Autodesk Inventor part; units mm, degrees
ref_plane "YZ Plane" through (0, 0, 0) normal (1, 0, 0) x (0, 1, 0)
ref_plane "XZ Plane" through (0, 0, 0) normal (0, 1, 0) x (-1, 0, 0)
ref_plane "XY Plane" through (0, 0, 0) normal (0, 0, 1) x (1, 0, 0)
sketch "Sketch1" plane through (0, 0, 0) normal (0, 1, 0) x (-1, 0, 0)
  circle A0 centre (0, 0) radius 3.175
  dimension "d0" = 6.35
extrude "Extrusion1" add sketch "Sketch1" along normal blind 31.75
sketch "Sketch2" plane through (0, 31.75, 0) normal (0, 1, 0) x (1, 0, 0)
  circle A0 centre (0, 0) radius 3.175
  circle A1 centre (0, 0) radius 4.7625
  dimension "d3" = 9.525
extrude "Extrusion2" add sketch "Sketch2" along normal blind 6.35 contours A0 | A1
sketch "Sketch3" plane through (0, 38.1, 0) normal (0, 1, 0) x (1, 0, 0)
  circle A0 centre (0, 0) radius 4.7625
  line L0 (-1.3748, 2.3812) -> (1.3748, 2.3813)
  line L1 (1.3748, 2.3813) -> (2.7496, 0)
  line L2 (2.7496, 0) -> (1.3748, -2.3813)
  line L3 (1.3748, -2.3813) -> (-1.3748, -2.3813)
  line L4 (-1.3748, -2.3813) -> (-2.7496, 0)
  line L5 (-2.7496, 0) -> (-1.3748, 2.3812)
  dimension "d6" = 4.7625
extrude "Extrusion3" cut sketch "Sketch3" against normal blind 3.175 contours L0 L1 L2 L3 L4 L5
fillet "Fillet1" radius 0.3969 3 edges at (3.175, 31.75, 0) (-4.7625, 38.1, 0) (3.175, 0, 0)
properties part number "Bolt_0.25_20_1.25len_SocketHead" material "Stainless Steel, Austenitic"
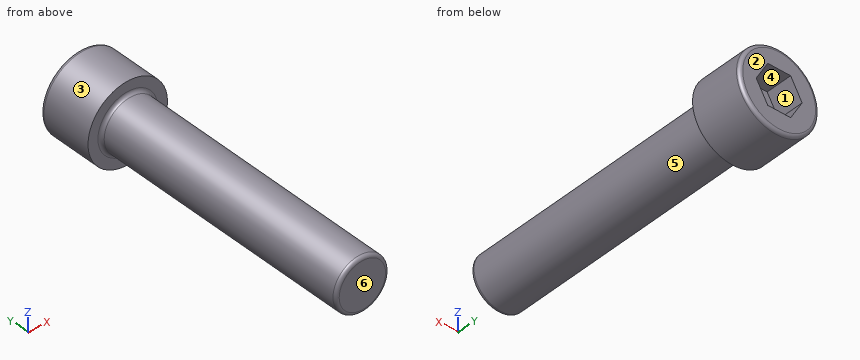
The listing builds one solid part. Answer for the finished solid, in the listing's coordinates (mm). Face numbers are marked on the shaded views. A direction names the side the tool comes from. Coordinates: 2 decimals unless noted, no trailing zeros. Loops run counter-clockwise (first coordinate to the right, second up) from the corner with the lowest first, then second, coordinate; pieces in that order, holes last. Notation, with made-up numbers: (5, 66.25) - (56, 66.25) arc R21 cw to (56, 70.25) - close; hole circle Ø11 at (-17.75, 85.25). An arc over 180 degrees is marked (long way). Write item = value, one per line.
1) Which of the six approach directions +Z, -Z, +X, -X, +Y, -Y give full straight-line access (tool end or side, diameter ignored) to the marked faces 5 and 6?
Responses:
face_5 = -Y
face_6 = +Z, -Z, +X, -X, -Y
2) Determine the mould class of the marked faces 1, 2, 3 and 4 for opening direction Z: pulls with the +Z half, pulls with the -Z half, needs draft (parallel to the pull), parting line crosses it, or undercut.
Responses:
face_1 = undercut
face_2 = needs draft
face_3 = parting line crosses it
face_4 = undercut
3) Section B-B (y = 24) is taken. Determine the outline of the cut face in (x, z) (3 decimals), plus the area to 3 significant figures.
Responses:
outline = circle Ø6.35 at (0, 0)
area = 31.7 mm^2
4) Each of these flat-tipped pins is pushed along its axis until it touches: P1, Ø1.4, axis at x = -0.5, z = 1, coming from the +Y side (3 decimals); P2, Ø1, axis at x = -0.5, y = 28, coming from the -Z side (3 decimals); P3, Ø2, axis at x = -1, y = 9, coming from the +Z side (3 decimals). Where does it stop, or does it pass through?
Responses:
P1 = 34.925
P2 = -3.175
P3 = 3.175
5) Find the intervals of material crossed by line 1 along Y through (x, z) = (-4, -1.75); line 2 along Y through (x, z) = (1.5, -0.5) (3 decimals); line 3 along X through (y, z) = (36, 1.75), in increasing order.
Responses:
line_1 = 31.75 to 38.1
line_2 = 0 to 34.925
line_3 = -4.43 to -1.74, 1.74 to 4.43
